```python
from build123d import *

# Parameters (mm, degrees)
BOX_W           = 25
BOX_H           = 22
BOX_DEPTH       = 26
SKETCH_R        = 8
POCKET_DEPTH    = 25.001
SKETCH001_R     = 3.5
POCKET001_DEPTH = 23
SKETCH002_R     = 1.8
POCKET002_DEPTH = 5
SKETCH003_R     = 1.8
POCKET003_DEPTH = 22.001
SKETCH004_W     = 2
SKETCH004_H     = 11.298807
SKETCH004_W_2   = 3
SKETCH004_H_2   = 8
POCKET004_DEPTH = 25.001


with BuildPart() as part:
    # Box → Box (new body)
    with BuildSketch(Plane.XY):
        with Locations((12.5, 11)):
            Rectangle(BOX_W, BOX_H)
    extrude(amount=BOX_DEPTH)

    # Sketch → Pocket (cut, through all)
    with BuildSketch(Plane.YZ.offset(25)):
        with Locations((11, 12.7)):
            Circle(SKETCH_R)
    extrude(amount=-POCKET_DEPTH, mode=Mode.SUBTRACT)

    # Sketch001 → Pocket001 (cut)
    with BuildSketch(Plane.XY.offset(26)):
        with Locations((7, 11)):
            Circle(SKETCH001_R)
        with Locations((18, 11)):
            Circle(SKETCH001_R)
    extrude(amount=-POCKET001_DEPTH, mode=Mode.SUBTRACT)

    # Sketch002 → Pocket002 (cut)
    with BuildSketch(Plane(origin=(0, 0, 0), x_dir=(1, 0, 0), z_dir=(0, 0, -1))):
        with Locations((7, -11)):
            Circle(SKETCH002_R)
        with Locations((18, -11)):
            Circle(SKETCH002_R)
    extrude(amount=-POCKET002_DEPTH, mode=Mode.SUBTRACT)

    # Sketch003 → Pocket003 (cut, through all)
    with BuildSketch(Plane(origin=(0, 22, 0), x_dir=(-1, 0, 0), z_dir=(0, 1, 0))):
        with Locations((-12.5, 22.5)):
            Circle(SKETCH003_R)
    extrude(amount=-POCKET003_DEPTH, mode=Mode.SUBTRACT)

    # Sketch004 → Pocket004 (cut, through all)
    with BuildSketch(Plane.YZ.offset(25)):
        with Locations((11, 23.747477)):
            Rectangle(SKETCH004_W, SKETCH004_H)
        with Locations((1.5, 22)):
            Rectangle(SKETCH004_W_2, SKETCH004_H_2)
        with Locations((20.5, 22)):
            Rectangle(SKETCH004_W_2, SKETCH004_H_2)
    extrude(amount=-POCKET004_DEPTH, mode=Mode.SUBTRACT)


solid = part.part
```
Here's how the part is built. I have some questions about the finished solid (model axes, mm). A direction names the side the tool comes from. Give positions to 0.01 mm unless a question says otherwise; leave off trailing zeros. Order: outer loops, then holes, each group sorted by start corner. A loop starts at its lowest first (then second) coordinate and runs counter-clockwise, first axis right, second up. Notation, with made-up numbers: (-30, -25) - (19, -25) arc R8 cw to (19, -21) - close; hole circle Ø9 at (28, 40). An arc over 180 degrees is marked (long way). Answer as a JSON object with one key per item and string values. Group by question number.
Item 1: If we section it at C-C on y = 13.75: Please give me the cut outline in (x, z).
Item 2: If we section it at B-B on z = 12.7: Please give me the cut outline in (x, y), and give its area (3 significant figures).
Item 3: If we section it at D-D on x = 12.5: Please give me the cut outline in (y, z).
Item 4: If we mould it in two halves opening along Z, with no side actions, what happens to faces 4 (the cylindrical face through (12.734, 15.549, 24.285)), 5 (the cylindrical face through (6.9, 7.5, 23)), 6 (the flat face through (12, 16, 26))? For each: pulls with the +Z half, pulls with the -Z half, needs draft (parallel to the pull), parting line crosses it, or undercut.
Item 5: If we section it at A-A on x = 7: Please give me the cut outline in (y, z).
Item 6: Which directions (+Z, -Z, +X, -X, +Y, -Y) give clear straight access to the entire face, cutting with the end or side of a thin tool? Please do faces 1 (the flat face through (23, 10, 23)), 2 (the cylindrical face through (14.503, 11.154, 3.992)), 3 (the flat face through (13, 20, 18)).
Item 7: Please list where these lines run through material, in increasing order: probe 1 along Y at (x, z) = (23.25, 23.5); probe 2 along Y at (x, z) = (12.75, 13); probe 3 along Z at (x, y) = (12.5, 8.5).
Item 8: For P1, Ø2, axis at x = 7, y = 11, coming from the +Z side; P2, Ø4, axis at x = 2, z = 23.5, coming from the -Y side; P3, Ø3, axis at x = 1, z = 23.5, coming from the +Y side; P4, Ø2, axis at x = 19, y = 10, coming from the +Z side, each with a flat end and sliding along its axis, tell me the tip position at first contact or that it passes through.
Result set:
{
 "1": {"outline": "(0, 0) - (25, 0) - (25, 5.19) - (20.17, 5.19) - (20.17, 3) - (15.83, 3) - (15.83, 5.19) - (9.17, 5.19) - (9.17, 3) - (4.83, 3) - (4.83, 5.19) - (0, 5.19) - close; (0, 20.21) - (4.83, 20.21) - (4.83, 26) - (0, 26) - close; (9.17, 20.21) - (15.83, 20.21) - (15.83, 26) - (9.17, 26) - close; (20.17, 20.21) - (25, 20.21) - (25, 26) - (20.17, 26) - close; hole circle Ø3.6 at (12.5, 22.5)"},
 "2": {"outline": "(0, 0) - (25, 0) - (25, 3) - (0, 3) - close; (0, 19) - (25, 19) - (25, 22) - (0, 22) - close", "area": "150 mm²"},
 "3": {"outline": "(0, 0) - (22, 0) - (22, 18) - (19, 18) - (19, 20.7) - (12, 20.7) - (12, 20.64) arc R8 cw (long way) to (10, 20.64) - (10, 20.7) - (3, 20.7) - (3, 18) - (0, 18) - close; (3, 24.3) - (10, 24.3) - (10, 26) - (3, 26) - close; (12, 24.3) - (19, 24.3) - (19, 26) - (12, 26) - close"},
 "4": {"face 4": "undercut", "face 5": "needs draft", "face 6": "pulls with the +Z half"},
 "5": {"outline": "(0, 0) - (9.2, 0) - (9.2, 3) - (7.5, 3) - (7.5, 5.51) arc R8 cw to (7.5, 19.89) - (7.5, 26) - (3, 26) - (3, 18) - (0, 18) - close; (12.8, 0) - (22, 0) - (22, 18) - (19, 18) - (19, 26) - (14.5, 26) - (14.5, 19.89) arc R8 cw to (14.5, 5.51) - (14.5, 3) - (12.8, 3) - close"},
 "6": {"face 1": "+Z, +X, -X", "face 2": "+Z", "face 3": "+Z, +X, -X, +Y"},
 "7": {"probe 1": "3 to 10, 12 to 19", "probe 2": "0 to 3.01, 18.99 to 22", "probe 3": "0 to 5.1, 20.3 to 20.7, 24.3 to 26"},
 "8": {"P1": "through", "P2": "y = 3", "P3": "y = 19", "P4": "z = 3"}
}
